Work out the finished part from the listing and answer in its coordinate system (mm). A direction names the side the tool comes from. Round coordinates to 2 decimals unless told otherwise and drop trailing zeros. Order: outer loops, then holes, each group sorted by start corner. A loop starts at its lowest first (then second) coordinate and runs counter-clockwise, first axis right, second up. Notation, with made-up numbers: (-3, 17.25) - (17, 17.25) arc R20 ccw to (17, 25.25) - close; hole circle Ø3 at (12, -23). An arc over 180 degrees is marked (long way). One line per question, with ' | ' between items. Start each with the question number.
from build123d import *

# Parameters (mm, degrees)
SKETCH_1_W          = 49
SKETCH_1_H          = 66
EXTRUDE_1_DEPTH     = 44
SKETCH_2_W          = 42
SKETCH_2_H          = 40
CUT_EXTRUDE_1_DEPTH = 42
SKETCH_3_W          = 20
SKETCH_3_H          = 24
CUT_EXTRUDE_2_DEPTH = 50
SKETCH_5_R          = 12
SKETCH_5_R_2        = 2.408268243
SKETCH_5_R_3        = 4.25
CUT_EXTRUDE_3_DEPTH = 50
SKETCH_7_R          = 5
CUT_EXTRUDE_4_DEPTH = 18
SKETCH_8_W          = 49
SKETCH_8_H          = 6
CUT_EXTRUDE_5_DEPTH = 18


with BuildPart() as part:
    # Sketch 1 → Extrude 1 (new body)
    with BuildSketch(Plane(origin=(0, 0, 0), x_dir=(1, 0, 0), z_dir=(0, 1, 0))):
        Rectangle(SKETCH_1_W, SKETCH_1_H)
    extrude(amount=EXTRUDE_1_DEPTH)

    # Sketch 2 → Cut-Extrude 1 (cut)
    with BuildSketch(Plane.XY.offset(33)):
        with Locations((0.48895233, 20)):
            Rectangle(SKETCH_2_W, SKETCH_2_H)
    extrude(amount=-CUT_EXTRUDE_1_DEPTH, mode=Mode.SUBTRACT)

    # Sketch 3 → Cut-Extrude 2 (cut)
    with BuildSketch(Plane.ZY.offset(24.5)):
        Polygon((-33, 24), (-13, 44), (-33, 44), align=None)
        with Locations((-23, 12)):
            Rectangle(SKETCH_3_W, SKETCH_3_H)
        Polygon((33, 0), (33, 44), (-13, 0), align=None)
    extrude(amount=-CUT_EXTRUDE_2_DEPTH, mode=Mode.SUBTRACT)

    # Sketch 5 → Cut-Extrude 3 (cut)
    with BuildSketch(Plane(origin=(0, 44, 0), x_dir=(1, 0, 0), z_dir=(0, 1, 0))):
        with Locations(Location((0, -14, 0), (0, 0, 270))):
            Circle(SKETCH_5_R)
        with Locations(Location((15.5, 1.5, 0), (0, 0, 270))):
            Circle(SKETCH_5_R_2)
        with Locations(Location((10.5, 23, 0), (0, 0, 270))):
            Circle(SKETCH_5_R_3)
        with Locations(Location((-10.5, 23, 0), (0, 0, 270))):
            Circle(SKETCH_5_R_3)
        with Locations(Location((15.5, -29.5, 0), (0, 0, 16.446238657))):
            Circle(SKETCH_5_R_2)
        with Locations(Location((-15.5, -29.5, 0), (0, 0, 270))):
            Circle(SKETCH_5_R_2)
        with Locations(Location((-15.5, 1.5, 0), (0, 0, 90))):
            Circle(SKETCH_5_R_2)
    extrude(amount=-CUT_EXTRUDE_3_DEPTH, mode=Mode.SUBTRACT)

    # Sketch 7 → Cut-Extrude 4 (cut)
    with BuildSketch(Plane(origin=(0, 44, 0), x_dir=(1, 0, 0), z_dir=(0, 1, 0))):
        with Locations(Location((10.5, 23, 0), (0, 0, 270))):
            Circle(SKETCH_7_R)
        with Locations(Location((-10.5, 23, 0), (0, 0, 270))):
            Circle(SKETCH_7_R)
    extrude(amount=-CUT_EXTRUDE_4_DEPTH, mode=Mode.SUBTRACT)

    # Sketch 8 → Cut-Extrude 5 (cut)
    with BuildSketch(Plane(origin=(0, 0, -13), x_dir=(-1, 0, 0), z_dir=(0, 0, -1))):
        with Locations((0, 3)):
            Rectangle(SKETCH_8_W, SKETCH_8_H)
    extrude(amount=-CUT_EXTRUDE_5_DEPTH, mode=Mode.SUBTRACT)


solid = part.part
1) Section B-B on x = 10.5 is taken. Give the vertices of the cut face in (y, z), and give its area (3 significant figures).
2) For faces 1 (the cylindrical face through (0.53, 42.03, 2.01)), 2 (the flat face through (8, 26, -27)), 3 (the flat face through (0, 24, -23)), 4 (the flat face through (-20.511, 27, 2)), determine the directions among +Z, -Z, +X, -X, +Y, -Y from which every point of the face is accessible in a straight line to the end or side of a thin tool.
3) Straight lines are drawn through the part: line 1 (X direction, y = 29.5, z = -23); line 2 (X direction, y = 41.75, z = -1.5); line 3 (X direction, y = 36, z = 12). For each, find the intervals that lie inside material, in ascending order.
4) Section A-A on z = -1.5 is taken. Give the vertices of the cut face in (x, y), and give its area (3 significant figures).
5) Determine the mould class of faces 5 (the flat face through (0, 15, -13)), 6 (the flat face through (21.489, 27, 2)), 7 (the flat face through (-13, 26, -27)), 8 (the flat face through (-1.929, 40.57, 29.414)) for opening direction Z: released by +Z, released by -Z, zero draft, split by the parting line, or undercut.
6) Section D-D on z = 14 is taken. Give the vertices of the cut face in (x, y).
7) Section C-C on y = 16.5 is taken. Give the vertices of the cut face in (x, z), and give its area (3 significant figures).
8) Flat-ended cylindrical pins translate along their axes: pin 1 (4 mm diameter, centred on x = 14.5, z = -2.5, fed in from +Y); pin 2 (9 mm diameter, centred on x = -10.5, z = -23, fed in from -Y); pin 3 (14.5 mm diameter, centred on x = 0, z = 14, fed in from +Y); pin 4 (7.5 mm diameter, centred on x = -15.5, z = -1.5, fed in from -Y). Find the tip coordinate at first contact, or state that the pin passes through.
Recorded:
1) outline: (6, -13) - (24, -13) - (24, -18.75) - (26, -18.75) - (26, -18) - (39, -18) - (44, -13) - (44, 8.19) - (40, 8.19) - (40, -9) - (6, -9) - close; (24, -33) - (29, -28) - (26, -28) - (26, -27.25) - (24, -27.25) - close; (40, 19.81) - (44, 19.81) - (44, 33) - (40, 28.82) - close | area: 368 mm²
2) face 1: +Y, -Y | face 2: +Y | face 3: -Z, +X, -X, -Y | face 4: +Z, -Y
3) line 1: x = -24.5 to -15.5, -5.5 to 5.5, 15.5 to 24.5 | line 2: x = -24.5 to -17.91, -13.09 to 13.09, 17.91 to 24.5 | line 3: x = -24.5 to -20.51, 21.49 to 24.5
4) outline: (-24.5, 11) - (-20.51, 11) - (-20.51, 40) - (-17.91, 40) - (-17.91, 44) - (-24.5, 44) - close; (-13.09, 40) - (13.09, 40) - (13.09, 44) - (-13.09, 44) - close; (17.91, 40) - (21.49, 40) - (21.49, 11) - (24.5, 11) - (24.5, 44) - (17.91, 44) - close | area: 360 mm²
5) face 5: released by -Z | face 6: zero draft | face 7: undercut | face 8: released by +Z
6) outline: (-24.5, 25.83) - (-20.51, 25.83) - (-20.51, 40) - (-12, 40) - (-12, 44) - (-24.5, 44) - close; (12, 40) - (21.49, 40) - (21.49, 25.83) - (24.5, 25.83) - (24.5, 44) - (12, 44) - close
7) outline: (-24.5, -13) - (24.5, -13) - (24.5, 4.25) - (21.49, 4.25) - (21.49, -9) - (-20.51, -9) - (-20.51, 4.25) - (-24.5, 4.25) - close | area: 289 mm²
8) pin 1: stops at y = 44 | pin 2: stops at y = 24 | pin 3: passes through | pin 4: stops at y = 40
